```python
from build123d import *

# Parameters (mm, degrees)
SKETCH019_R     = 4.25
PAD010_DEPTH    = 5
PAD009_DEPTH    = 3
SKETCH021_R     = 8.625
POCKET008_DEPTH = 3
POCKET009_DEPTH = 3
SKETCH018_R     = 1.6
POCKET007_DEPTH = 8.001
SKETCH022_R     = 1.6
PAD011_DEPTH    = 3
FILLET020_R     = 0.35
FILLET021_R     = 0.35
FILLET022_R     = 0.25
FILLET023_R     = 1.3
FILLET024_R     = 1.3


with BuildPart() as part:
    # Sketch019 → Pad010 (new body)
    with BuildSketch(Plane.XY):
        Polygon((-3, 6.9), (15, 6.9), (46.204036, -1.461096), (52, -11.5), (52, -24.8), (8.85, -24.8), (-6.05, -9.9), (-6.05, 3.85), align=None)
        with Locations((32.65, -11.5)):
            Circle(SKETCH019_R, mode=Mode.SUBTRACT)
    extrude(amount=PAD010_DEPTH)

    # Sketch020 → Pad009 (join)
    with BuildSketch(Plane.XY):
        Polygon((0.3, -16.25), (13.9, -16.25), (13.9, -24.8), (8.85, -24.8), align=None)
    extrude(amount=-PAD009_DEPTH)

    # Sketch021 → Pocket008 (cut)
    with BuildSketch(Plane.XY.offset(5)):
        with Locations((32.65, -11.5)):
            Circle(SKETCH021_R)
    extrude(amount=-POCKET008_DEPTH, mode=Mode.SUBTRACT)

    # Sketch017 → Pocket009 (cut)
    with BuildSketch(Plane.XY.offset(5)):
        Polygon((0, -3.5), (3.031089, -1.75), (3.031089, 1.75), (0, 3.5), (-3.031089, 1.75), (-3.031089, -1.75), align=None)
    extrude(amount=-POCKET009_DEPTH, mode=Mode.SUBTRACT)

    # Sketch018 → Pocket007 (cut, through all)
    with BuildSketch(Plane.XY.offset(-3)):
        Circle(SKETCH018_R)
    extrude(amount=POCKET007_DEPTH, mode=Mode.SUBTRACT)

    # Sketch022 → Pad011 (join)
    with BuildSketch(Plane.XY):
        Polygon((0, -3.15), (2.72798, -1.575), (2.72798, 1.575), (0, 3.15), (-2.72798, 1.575), (-2.72798, -1.575), align=None)
        Circle(SKETCH022_R, mode=Mode.SUBTRACT)
    extrude(amount=-PAD011_DEPTH)

    # Fillet020
    fillet020_edges = [part.edges().sort_by_distance(p)[0] for p in [
        (-1.515544, -2.625, 5),
        (-3.031089, 0, 5),
        (-1.515544, 2.625, 5),
        (1.515544, 2.625, 5),
        (3.031089, 0, 5),
        (1.515544, -2.625, 5),
    ]]
    fillet(fillet020_edges, radius=FILLET020_R)

    # Fillet021
    fillet021_edges = [part.edges().sort_by_distance(p)[0] for p in [
        (24.025, -11.5, 5),
    ]]
    fillet(fillet021_edges, radius=FILLET021_R)

    # Fillet022
    fillet022_edges = [part.edges().sort_by_distance(p)[0] for p in [
        (1.36399, -2.3625, -3),
        (2.72798, 0, -3),
        (1.36399, 2.3625, -3),
        (-1.36399, 2.3625, -3),
        (-2.72798, 0, -3),
        (-1.36399, -2.3625, -3),
        (-1.6, 0, -3),
    ]]
    fillet(fillet022_edges, radius=FILLET022_R)

    # Fillet023
    fillet023_edges = [part.edges().sort_by_distance(p)[0] for p in [
        (7.1, -16.25, -3),
        (13.9, -20.525, -3),
        (11.375, -24.8, -3),
        (4.575, -20.525, -3),
    ]]
    fillet(fillet023_edges, radius=FILLET023_R)

    # Fillet024
    fillet024_edges = [part.edges().sort_by_distance(p)[0] for p in [
        (52, -18.15, 5),
        (30.425, -24.8, 5),
        (1.4, -17.35, 5),
        (-6.05, -3.025, 5),
        (-4.525, 5.375, 5),
        (6, 6.9, 5),
        (30.602018, 2.719452, 5),
        (49.102018, -6.480548, 5),
    ]]
    fillet(fillet024_edges, radius=FILLET024_R)


with BuildPart() as part_1:
    # Body003 placement: moved
    add(part.part.moved(Location((2.25, -88, 0))))


solid = part_1.part
```
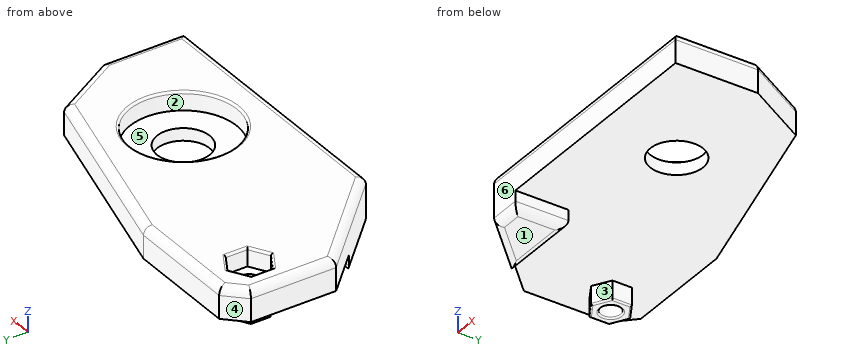
Build history of the part. All positions in model axes, mm. Face numbers are marked on the shaded views. A direction names the side the tool comes from. Round coordinates to 2 decimals unless told otherwise and drop trailing zeros. Write each loop counter-clockwise with the first axis right and the second up, starting at its lowest first coordinate (ties: lowest second). Pieces come first, ordered by that corner, then holes. Notation, with made-up numbers: (-6.75, -25.75) - (47.25, -25.75) arc R13 ccw to (47.25, -7.75) - close; hole circle Ø8 at (66.5, 38). An arc over 180 degrees is marked (long way). Answer as CSV lines item,"result".
Q1. Pull direction Y, two halves, no side cores. Call the marked faces 3, 4, 5 and 6: +Y half, -Y half, draft (parallel to the pull), parting line (faces both ways), or undercut.
Report:
face 3,"undercut"
face 4,"+Y half"
face 5,"undercut"
face 6,"-Y half"
Q2. Drop flat-ended pins along their axis: pin 1 (0.8 mm diameter, centred on x = 7, z = -0.5, fed in from +Y); pin 2 (16 mm diameter, centred on x = 30, y = -92, fed in from -Z); pin 3 (5 mm diameter, centred on x = 32.5, y = -100.5, fed in from +Z); pin 4 (7 mm diameter, centred on x = 34.9, y = -99.5, fed in from -Z). Give the stop position or say it passes through.
Report:
pin 1,"stops at y = -104.25"
pin 2,"stops at z = 0"
pin 3,"stops at z = 2"
pin 4,"passes through"
Q3. Tool access for the marked faces 1 and 2: list every direction of +Z, -Z, +X, -X, +Y, -Y with a clear straight run to the whole face (end or side of a thin tool).
Report:
face 1,"-Z, +X, -X, +Y, -Y"
face 2,"+Z"
Q4. Drill centre lines: probe 1 along Y at (x, z) = (2.25, -1.4); probe 2 along Z at (x, y) = (48.5, -105); probe 3 along Y at (x, z) = (2, 3). Where is each one in solid material? Low to high. Write a range as [from, to].
Report:
probe 1,"y = [-91.15, -89.6], [-86.4, -84.85]"
probe 2,"z = [0, 5]"
probe 3,"y = [-103.7, -91.36], [-84.64, -81.1]"
Q5. Cut at A-A (x = 13). Write the cut outline in (y, z).
Report:
outline,"(-112.8, -1.7) arc R1.3 ccw to (-111.5, -3) - (-105.55, -3) arc R1.3 ccw to (-104.25, -1.7) - (-104.25, 0) - (-81.1, 0) - (-81.1, 3.7) arc R1.3 ccw to (-82.4, 5) - (-111.5, 5) arc R1.3 ccw to (-112.8, 3.7) - close"
